Read the model definition and answer for the solid it produces. Units are mm, in the model's axes. Face numbers are marked on the shaded views. A direction names the side the tool comes from. Give positions to 0.01 mm unless a question says otherwise; leave off trailing zeros. Order: outer loops, then holes, each group sorted by start corner. A loop starts at its lowest first (then second) coordinate and runs counter-clockwise, first axis right, second up.
```python
from build123d import *

# Parameters (mm, degrees)
F0_W     = 50.8
F0_H     = 76.2
F0_W_2   = 44.45
F0_H_2   = 69.85
F2_DEPTH = 311.15
F3_R     = 3.175
F4_R     = 3
F5_DEPTH = 25.4
F6_DEPTH = 25.4


# Not quite as in the source:
# - a variable given as a bare number and used for a length is read in inches; the dataset says mm whatever the document's units were


with BuildPart() as f2:
    # F0 (on Right) → F2 (new body)
    with BuildSketch(Plane.YZ):
        Rectangle(F0_W, F0_H)
        Rectangle(F0_W_2, F0_H_2, mode=Mode.SUBTRACT)
    extrude(amount=F2_DEPTH)

    # F3
    f3_edges = [f2.edges().sort_by_distance(p)[0] for p in [
        (155.575, -25.4, 38.1),
        (155.575, -22.225, 34.925),
        (155.575, 22.225, 34.925),
        (155.575, 25.4, 38.1),
        (155.575, 25.4, -38.1),
        (155.575, -25.4, -38.1),
        (155.575, 22.225, -34.925),
        (155.575, -22.225, -34.925),
    ]]
    fillet(f3_edges, radius=F3_R)

    # F4 (on face) → F5 (cut)
    with BuildSketch(Plane.XZ.offset(25.4)):
        with Locations((37.975, 15)):
            Circle(F4_R)
        with Locations((69.975, 15)):
            Circle(F4_R)
        with Locations((69.975, -15)):
            Circle(F4_R)
        with Locations((37.975, -15)):
            Circle(F4_R)
        with Locations((241.175, 15)):
            Circle(F4_R)
        with Locations((273.175, 15)):
            Circle(F4_R)
        with Locations((273.175, -15)):
            Circle(F4_R)
        with Locations((241.175, -15)):
            Circle(F4_R)
    extrude(amount=-F5_DEPTH, mode=Mode.SUBTRACT)

    # F4 (on face) → F6 (cut)
    with BuildSketch(Plane.XZ.offset(25.4)):
        with Locations((117.475, 12.7)):
            Circle(F4_R)
        with Locations((117.475, -12.7)):
            Circle(F4_R)
        with Locations((193.675, -12.7)):
            Circle(F4_R)
        with Locations((193.675, 12.7)):
            Circle(F4_R)
    extrude(amount=-F6_DEPTH, mode=Mode.SUBTRACT)


solid = f2.part
```
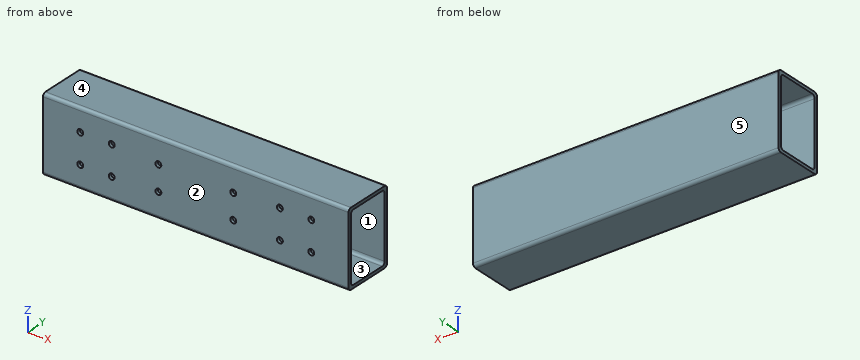
1) A tool of negligible diameter and unlimited length cuts with its end or side. For the marked faces 1 and 2, from which of +Z, -Z, +X, -X, +Y, -Y can it reach the whole face along a straight path? Write none if from no direction.
Final values:
face 1: +X, -X
face 2: +Z, -Z, +X, -X, -Y
2) Given pin 1 (5 mm diameter, centred on x = 69.975, z = -15, fed in from -Y) (3 decimals); pin 2 (9.5 mm diameter, centred on x = 241.175, z = -15, fed in from -Y), each flat-ended and moving along its own axis, determine where each tip first touches the part or whether it passes through.
Final values:
pin 1: stops at y = 22.225
pin 2: stops at y = -25.4
3) The part is cut by section B-B on x = 161. Determine the outline of the cut face in (y, z) (3 decimals).
Final values:
outline: (-25.4, -34.925) arc R3.175 ccw to (-22.225, -38.1) - (22.225, -38.1) arc R3.175 ccw to (25.4, -34.925) - (25.4, 34.925) arc R3.175 ccw to (22.225, 38.1) - (-22.225, 38.1) arc R3.175 ccw to (-25.4, 34.925) - close; hole (-22.225, -31.75) arc R3.175 ccw to (-19.05, -34.925) - (19.05, -34.925) arc R3.175 ccw to (22.225, -31.75) - (22.225, 31.75) arc R3.175 ccw to (19.05, 34.925) - (-19.05, 34.925) arc R3.175 ccw to (-22.225, 31.75) - close
4) For a pull along Z with two mould halves and no side action, classify the marked faces 3, 4 and 5 as released by +Z, released by -Z, zero draft, split by the parting line, or undercut.
Final values:
face 3: undercut
face 4: released by +Z
face 5: zero draft
5) The part is cut by section A-A on y = 11.5. Determine the outline of the cut face in (x, z) (3 decimals), and give its area (3 significant figures).
Final values:
outline: (0, -38.1) - (311.15, -38.1) - (311.15, -34.925) - (0, -34.925) - close; (0, 34.925) - (311.15, 34.925) - (311.15, 38.1) - (0, 38.1) - close
area: 1,980 mm2
6) Consider L1, parallel to Z at x = 256, y = 9.5 (3 decimals); L2, parallel to Y at x = 80, z = -5 (3 decimals); L3, parallel to Z at x = 242.5, y = -20. Determine where each line is inside the solid, lowest interval first.
Final values:
L1: z = -38.1 to -34.925, 34.925 to 38.1
L2: y = -25.4 to -22.225, 22.225 to 25.4
L3: z = -38.1 to -34.78, 34.78 to 38.1
